For this review, use the dimensioned drawing (mm, ordinates from the lowest corner) and the shaded views. Coordinates: 2 decimals unless noted, no trailing zeros. Order: outer loops, then holes, each group sorted by start corner. A loop starts at its lowest first (then second) coordinate and runs counter-clockwise, first axis right, second up. Notation, with made-up numbers: M -18.75,-10 L -1.75,-10 A14 cw -1.75,1 Z; hole C -30,65 d7. An arc over 180 degrees is marked long. Answer in a Markdown table with one row per item.
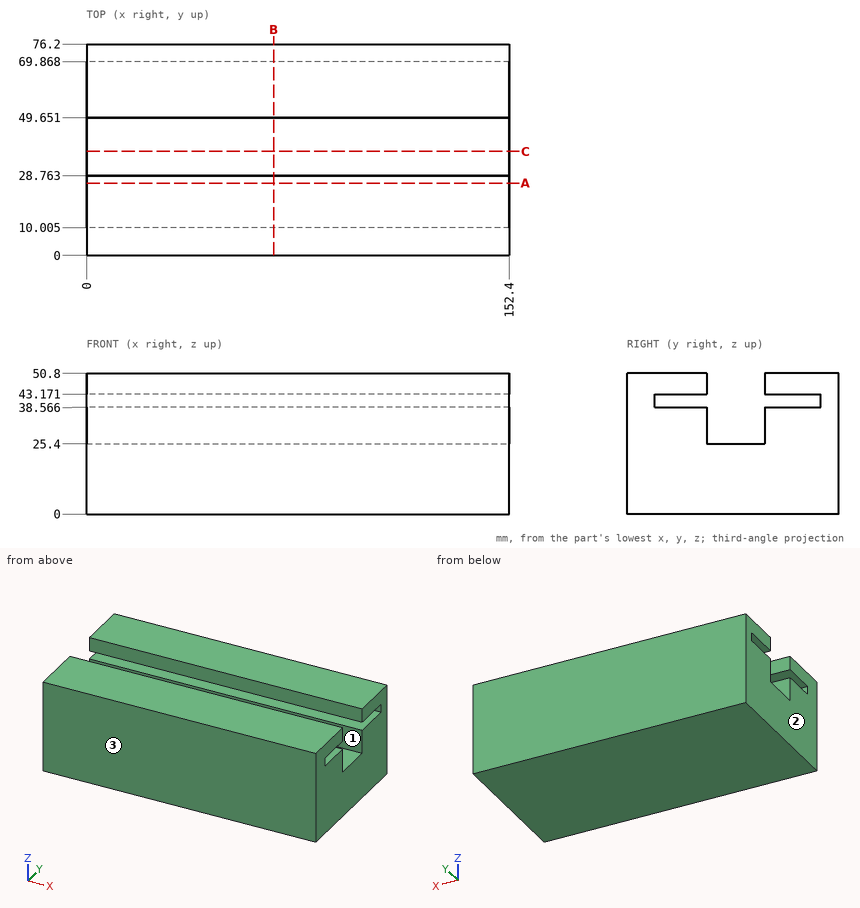
(1) For line 1 along Y through (x, z) = (32.5, 31); line 2 along Z through (x, y) = (116.5, 19); line 3 along Y through (x, z) = (12, 43) (1 decimal), list the stretches that pass through material, from the lowest coordinate up. Write a range as from..to.
Return value:
| item | result |
|---|---|
| line 1 | y = 0..28.76, 49.65..76.2 |
| line 2 | z = 0..38.57, 43.17..50.8 |
| line 3 | y = 0..10, 69.9..76.2 |
(2) Add section B-B, the plane x = 67.5. Give the boundary of the cut face in (y, z) (1 decimal).
Return value:
| item | result |
|---|---|
| outline | M 0,0 L 76.2,0 L 76.2,50.8 L 49.7,50.8 L 49.7,43.2 L 69.9,43.2 L 69.9,38.6 L 49.7,38.6 L 49.7,25.4 L 28.8,25.4 L 28.8,38.6 L 10,38.6 L 10,43.2 L 28.8,43.2 L 28.8,50.8 L 0,50.8 Z |
(3) Draft analysis for pull direction Y (two halves, no side actions). For the marked faces 1, 2 and 3, state which applies: pulls with the +Y half, pulls with the -Y half, needs draft (parallel to the pull), parting line crosses it, or undercut.
Return value:
| item | result |
|---|---|
| face 1 | undercut |
| face 2 | needs draft |
| face 3 | pulls with the -Y half |
(4) Add section C-C, the plane y = 37.5. Give the boundary of the cut face in (x, z), and give its area (3 significant figures).
Return value:
| item | result |
|---|---|
| outline | M 0,0 L 152.4,0 L 152.4,25.4 L 0,25.4 Z |
| area | 3,870 mm2 |
(5) Insertion check: pin 1 Ø10.5 at (x, y) = (57, 42) entering from +Z. The pin has a flat end and moves straight along its axis. Give the tip position at first contact, or say it passes through.
Return value:
| item | result |
|---|---|
| pin 1 | stops at z = 25.4 |
(6) Add section A-A, the plane y = 26. Give the boundary of the cut face in (x, z).
Return value:
| item | result |
|---|---|
| outline | M 0,0 L 152.4,0 L 152.4,38.57 L 0,38.57 Z; M 0,43.17 L 152.4,43.17 L 152.4,50.8 L 0,50.8 Z |
